from build123d import *

# Parameters (mm, degrees)
CHAMFER1_SIZE      = 0.25
FILLET1_R          = 0.2
CUT_EXTRUDE1_DEPTH = 2
FILLET2_R          = 0.1


with BuildPart() as part:
    # Sketch1 → Revolve1 (revolve)
    with BuildSketch(Plane.XY):
        Polygon((0, -13), (-1.5, -13), (-1.5, -3), (-2.75, -3), (-2.75, 0), (0, 0), align=None)
    revolve(axis=Axis((0, 0, 0), (0, -1, 0)))

    # Chamfer1
    chamfer1_edges = [part.edges().sort_by_distance(p)[0] for p in [
        (1.5, -3, 0),
        (1.5, -13, 0),
    ]]
    chamfer(chamfer1_edges, length=CHAMFER1_SIZE)

    # Fillet1
    fillet1_edges = [part.edges().sort_by_distance(p)[0] for p in [
        (2.75, 0, 0),
    ]]
    fillet(fillet1_edges, radius=FILLET1_R)

    # Sketch2 → Cut-Extrude1 (cut)
    with BuildSketch(Plane(origin=(0, 0, 0), x_dir=(1, 0, 0), z_dir=(0, 1, 0))):
        Polygon((0, 1.443375673), (-1.25, 0.721687836), (-1.25, -0.721687836), (0, -1.443375673), (1.25, -0.721687836), (1.25, 0.721687836), align=None)
    extrude(amount=-CUT_EXTRUDE1_DEPTH, mode=Mode.SUBTRACT)

    # Fillet2
    fillet2_edges = [part.edges().sort_by_distance(p)[0] for p in [
        (0.625, -2, -1.082531755),
        (1.25, -2, 0),
        (0.625, -2, 1.082531755),
        (-0.625, -2, 1.082531755),
        (-1.25, -2, 0),
        (-0.625, -2, -1.082531755),
        (0.625, 0, -1.082531755),
        (-0.625, 0, -1.082531755),
        (-1.25, 0, 0),
        (-0.625, 0, 1.082531755),
        (0.625, 0, 1.082531755),
        (1.25, 0, 0),
    ]]
    fillet(fillet2_edges, radius=FILLET2_R)


solid = part.part
The model under review builds one solid part; all positions refer to its coordinate system, in mm. A direction names the side the tool comes from. Coordinates: 2 decimals unless noted, no trailing zeros. Loops run counter-clockwise (first coordinate to the right, second up) from the corner with the lowest first, then second, coordinate; pieces in that order, holes last.
(1) Insertion check: P1, Ø1.8, axis at x = 0.5, z = -0.5, coming from the +Y side. The pin has a flat end and moves straight along its axis. Give the tip position at first contact, or say it passes through.
Determined:
P1: stops at y = 0
(2) Tool access review of faces 5 (the flat face through (0.63, -0.99, -1.08)), 6 (the flat face through (-1.1, 0, 1.1)), 7 (the flat face through (2, -3, 0)): name each direction out of +Z, -Z, +X, -X, +Y, -Y from which nothing blocks a thin tool from reaching the whole face with its end or side.
Determined:
face 5: +Y
face 6: +Z, -Z, +X, -X, +Y
face 7: -Y
(3) Draft analysis for pull direction Z (two halves, no side actions). For faces 1 (the flat face through (0.616, -0.987, 1.088)), 2 (the flat face through (0, -13, 0)), 3 (the cylindrical face through (1.5, -7.93, -0.07)), 4 (the flat face through (1.25, -1, 0)), state which applies: +Z half, -Z half, draft (parallel to the pull), parting line (faces both ways), or undercut.
Determined:
face 1: undercut
face 2: draft
face 3: parting line
face 4: undercut
(4) Wall thickness on L1, parallel to X at y = -5.5, z = 0.1; L2, parallel to Y at x = -2.5, z = 0.6; L3, parallel to Z at x = -0.6, y = -0.25: over which ranges is each line inside the solid? List them lowest first.
Determined:
L1: x = -1.5 to 1.5
L2: y = -3 to 0
L3: z = -2.68 to -1.1, 1.1 to 2.68
(5) Consider section B-B, the plane y = -7.75. Give the boundary of the cut face in (x, z), plus the area to 3 significant figures.
Determined:
outline: circle Ø3 at (0, 0)
area: 7.07 mm2
(6) Consider section A-A, the plane z = 0. Give the boundary of the cut face in (x, y).
Determined:
outline: (-2.75, -3) - (-1.75, -3) - (-1.5, -3.25) - (-1.5, -12.75) - (-1.25, -13) - (1.25, -13) - (1.5, -12.75) - (1.5, -3.25) - (1.75, -3) - (2.75, -3) - (2.75, -0.2) arc R0.2 ccw to (2.55, 0) - (1.35, 0) arc R0.1 ccw to (1.25, -0.1) - (1.25, -1.9) arc R0.1 cw to (1.15, -2) - (-1.15, -2) arc R0.1 cw to (-1.25, -1.9) - (-1.25, -0.1) arc R0.1 ccw to (-1.35, 0) - (-2.55, 0) arc R0.2 ccw to (-2.75, -0.2) - close
